Geometry: see drawing. Coordinates: mm, zero at the bounding-box minimum. Give positions to 0.01 mm unless a question says otherwise; leave off trailing zeros. Loops run counter-clockwise (first coordinate to the right, second up) from the corner with the lowest first, then second, coordinate; pieces in that order, holes last. Notation, with made-up numbers: M 25.25,58 L 36.25,58 A29 ccw 36.25,89 Z; hole C 52.25,86.5 d1. An arc over 180 degrees is marked long. Answer in a Markdown table with one row per item.
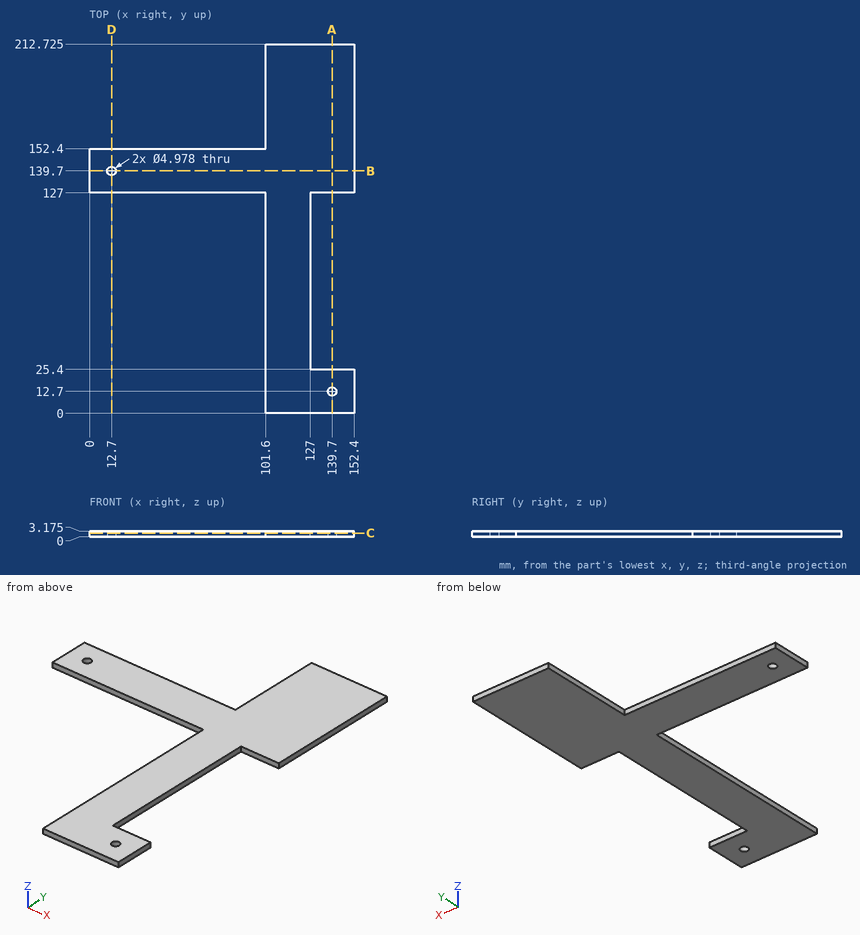
1) Section D-D, the plane x = 12.7. Return loops of the section in (y, z) (1 decimal).
Reply:
| item | result |
|---|---|
| outline | M 127,0 L 137.2,0 L 137.2,3.2 L 127,3.2 Z; M 142.2,0 L 152.4,0 L 152.4,3.2 L 142.2,3.2 Z |
2) Pin query (flat end, axial travel): pin 1 Ø1.6 at (x, z) = (48.5, 1) entering from -Y; pin 2 Ø1.6 at (y, z) = (190.5, 1) entering from -X; pin 3 Ø1.6 at (x, z) = (58, 1.5) entering from +Y. Return the tip coordinate at first contact, or that it passes through.
Reply:
| item | result |
|---|---|
| pin 1 | stops at y = 127 |
| pin 2 | stops at x = 101.6 |
| pin 3 | stops at y = 152.4 |
3) Material intervals for L1, parallel to Y at x = 139.7, z = 2.1 (1 decimal); L2, parallel to Y at x = 132, z = 2.6 (1 decimal); L3, parallel to X at y = 139.7, z = 1.5, sorted ascending.
Reply:
| item | result |
|---|---|
| L1 | y = 0 to 10.2, 15.2 to 25.4, 127 to 212.7 |
| L2 | y = 0 to 25.4, 127 to 212.7 |
| L3 | x = 0 to 10.21, 15.19 to 152.4 |
4) Section B-B, the plane y = 139.7. Return loops of the section in (x, z) (1 decimal), then the cut area to 3 significant figures.
Reply:
| item | result |
|---|---|
| outline | M 0,0 L 10.2,0 L 10.2,3.2 L 0,3.2 Z; M 15.2,0 L 152.4,0 L 152.4,3.2 L 15.2,3.2 Z |
| area | 468 mm² |
5) Section A-A, the plane x = 139.7. Return loops of the section in (y, z) (1 decimal).
Reply:
| item | result |
|---|---|
| outline | M 0,0 L 10.2,0 L 10.2,3.2 L 0,3.2 Z; M 15.2,0 L 25.4,0 L 25.4,3.2 L 15.2,3.2 Z; M 127,0 L 212.7,0 L 212.7,3.2 L 127,3.2 Z |
6) Section C-C, the plane z = 2.2. Return loops of the section in (x, y) (1 decimal).
Reply:
| item | result |
|---|---|
| outline | M 0,127 L 101.6,127 L 101.6,0 L 152.4,0 L 152.4,25.4 L 127,25.4 L 127,127 L 152.4,127 L 152.4,212.7 L 101.6,212.7 L 101.6,152.4 L 0,152.4 Z; hole C 12.7,139.7 d5; hole C 139.7,12.7 d5 |
